from build123d import *

# Parameters (mm, degrees)
SKETCH2_W           = 55
SKETCH2_H           = 93
BOSS_EXTRUDE1_DEPTH = 3
SKETCH3_W           = 10.997747865
SKETCH3_H           = 9.016820523
CUT_EXTRUDE1_DEPTH  = 3


with BuildPart() as part:
    # Sketch2 → Boss-Extrude1 (new body)
    with BuildSketch(Plane(origin=(0, 0, 0), x_dir=(0, 0, -1), z_dir=(1, 0, 0))):
        Rectangle(SKETCH2_W, SKETCH2_H)
    extrude(amount=BOSS_EXTRUDE1_DEPTH)

    # Sketch3 → Cut-Extrude1 (cut)
    with BuildSketch(Plane(origin=(3, 0, 0), x_dir=(0, 0, -1), z_dir=(1, 0, 0))):
        Polygon((-27.5, 46.5), (-24.5, 46.5), (-15, 46.5), (-15, 43.5), (-24.5, 43.5), (-24.5, 10), (-27.5, 10), align=None)
        Polygon((27.5, 46.5), (27.5, 10), (24.5, 10), (24.5, 43.5), (15, 43.5), (15, 46.5), (24.5, 46.5), align=None)
        Polygon((27.5, -46.5), (24.5, -46.5), (15, -46.5), (15, -43.5), (24.5, -43.5), (24.5, -10), (27.5, -10), align=None)
        Polygon((-27.5, -46.5), (-27.5, -10), (-24.5, -10), (-24.5, -43.5), (-15, -43.5), (-15, -46.5), (-24.5, -46.5), align=None)
        with Locations((-12.014032646, -34.210673658)):
            Rectangle(SKETCH3_W, SKETCH3_H)
    extrude(amount=-CUT_EXTRUDE1_DEPTH, mode=Mode.SUBTRACT)


solid = part.part
Work out the finished part from the listing and answer in its coordinate system (mm). A direction names the side the tool comes from. Give positions to 0.01 mm unless a question says otherwise; leave off trailing zeros. Write each loop counter-clockwise with the first axis right and the second up, starting at its lowest first coordinate (ties: lowest second). Pieces come first, ordered by that corner, then holes.
Q1. Given pin 1 (0.9 mm diameter, centred on x = 1, y = -35.5, fed in from +Z); pin 2 (0.9 mm diameter, centred on x = 1, z = -26, fed in from -Y); pin 3 (1.5 mm diameter, centred on x = 2, y = -45.5, fed in from -Z), each flat-ended and moving along its own axis, determine where each tip first touches the part or whether it passes through.
Answer:
pin 1: stops at z = 24.5
pin 2: stops at y = -10
pin 3: stops at z = -15
Q2. The part is cut by section A-A on z = 14. Give the vertices of the cut face in (x, y), and give its area (3 significant figures).
Answer:
outline: (0, -46.5) - (3, -46.5) - (3, -38.72) - (0, -38.72) - close; (0, -29.7) - (3, -29.7) - (3, 46.5) - (0, 46.5) - close
area: 252 mm2
Q3. A tool of negligible diameter and unlimited length cuts with its end or side. For faces 5 (the face through (2, -38.719, 12)), 6 (the face through (2, 45, -15)), 7 (the face through (2, 43.5, 20)), from which of +Z, -Z, +X, -X, +Y, -Y can it reach the whole face along a straight path? Write none if from no direction.
Answer:
face 5: +X, -X
face 6: -Z, +X, -X, +Y
face 7: +Z, +X, -X, +Y
Q4. The part is cut by section D-D on y = 14.5. Give the vertices of the cut face in (x, z).
Answer:
outline: (0, -24.5) - (3, -24.5) - (3, 24.5) - (0, 24.5) - close
Q5. For a pull along Y with two mould halves and no side action, classify faces 1 (the face through (2, -43.5, -20)), 2 (the face through (2, -45, 15)), 3 (the face through (2, 43.5, -20)), 4 (the face through (2, -34, 17.513)) as released by +Y, released by -Y, zero draft, split by the parting line, or undercut.
Answer:
face 1: released by -Y
face 2: zero draft
face 3: released by +Y
face 4: undercut
Q6. Straight lines are drawn through the part: L1, parallel to Y at x = 1.8, z = 10.5; L2, parallel to Z at x = 1.05, y = 37.5; L3, parallel to Z at x = 2.1, y = -38. For each, find the intervals that lie inside material, in ascending order.
Answer:
L1: y = -46.5 to -38.72, -29.7 to 46.5
L2: z = -24.5 to 24.5
L3: z = -24.5 to 6.52, 17.51 to 24.5
Q7. The part is cut by section B-B on y = -31. Give the vertices of the cut face in (x, z), and give its area (3 significant figures).
Answer:
outline: (0, -24.5) - (3, -24.5) - (3, 6.52) - (0, 6.52) - close; (0, 17.51) - (3, 17.51) - (3, 24.5) - (0, 24.5) - close
area: 114 mm2
Q8. The part is cut by section C-C on x = 0.65. Give the vertices of the cut face in (y, z), and give its area (3 significant figures).
Answer:
outline: (-46.5, -15) - (-43.5, -15) - (-43.5, -24.5) - (-10, -24.5) - (-10, -27.5) - (10, -27.5) - (10, -24.5) - (43.5, -24.5) - (43.5, -15) - (46.5, -15) - (46.5, 15) - (43.5, 15) - (43.5, 24.5) - (10, 24.5) - (10, 27.5) - (-10, 27.5) - (-10, 24.5) - (-43.5, 24.5) - (-43.5, 15) - (-46.5, 15) - close; hole (-38.72, 6.52) - (-29.7, 6.52) - (-29.7, 17.51) - (-38.72, 17.51) - close
area: 4,460 mm2
